Verification items for the finished model (mm, model axes). A direction names the side the tool comes from. Coordinates: 2 decimals unless noted, no trailing zeros. Write item = value, one per line.
```python
from build123d import *

# Parameters (mm, degrees)
SKETCH_1_R           = 1.5
SKETCH_1_R_2         = 17.5
SKETCH_1_R_3         = 12
SKETCH_1_R_4         = 1.25
EXTRUDE_1_DEPTH      = 4
SKETCH_2_R           = 18.5
SKETCH_2_R_2         = 17.5
CUT_EXTRUDE_1_DEPTH  = 3
SKETCH_3_W           = 10
SKETCH_3_H           = 5
SKETCH_3_W_2         = 6
CUT_EXTRUDE_2_DEPTH  = 93.020070098
CUT_EXTRUDE_3_DEPTH  = 93.020070098
FILLET_2_R           = 2
SKETCH_6_R           = 1.25
CUT_EXTRUDE_5_DEPTH  = 10
SKETCH_7_R           = 1.65
CUT_EXTRUDE_6_DEPTH  = 10
SKETCH_9_R           = 1.65
CUT_EXTRUDE_7_DEPTH  = 10
SKETCH_10_R          = 17.5
SKETCH_10_R_2        = 10.270750689
CUT_EXTRUDE_8_DEPTH  = 2
SKETCH_11_R          = 1.5
CUT_EXTRUDE_9_DEPTH  = 10
SKETCH_12_R          = 1.525
CUT_EXTRUDE_10_DEPTH = 10


with BuildPart() as part:
    # 草图1 → 凸台-拉伸1 (new body)
    with BuildSketch(Plane.XY):
        with BuildLine():
            Line((-27.534883443, -40.634933888), (42.465116557, -40.634933888))
            ThreePointArc((42.465116557, -40.634933888), (48.890398145, -38.615583047), (55.528781273, -37.478089862))
            ThreePointArc((55.528781273, -37.478089862), (82.425879892, -6.10109544), (52.465116557, 22.365066112))
            Line((52.465116557, 22.365066112), (-37.534883443, 22.365066112))
            ThreePointArc((-37.534883443, 22.365066112), (-67.495646778, -6.10109544), (-40.598548158, -37.478089862))
            ThreePointArc((-40.598548158, -37.478089862), (-33.960165031, -38.615583047), (-27.534883443, -40.634933888))
        make_face()
        with Locations((52.465116557, 13.115066112)):
            Circle(SKETCH_1_R, mode=Mode.SUBTRACT)
        with Locations((67.137582267, 7.037531822)):
            Circle(SKETCH_1_R, mode=Mode.SUBTRACT)
        with Locations((73.215116557, -7.634933888)):
            Circle(SKETCH_1_R, mode=Mode.SUBTRACT)
        with Locations((67.137582267, -22.307399597)):
            Circle(SKETCH_1_R, mode=Mode.SUBTRACT)
        with Locations((52.465116557, -28.384933888)):
            Circle(SKETCH_1_R, mode=Mode.SUBTRACT)
        with Locations((37.792650848, -22.307399597)):
            Circle(SKETCH_1_R, mode=Mode.SUBTRACT)
        with Locations((31.715116557, -7.634933888)):
            Circle(SKETCH_1_R, mode=Mode.SUBTRACT)
        with Locations((37.792650848, 7.037531822)):
            Circle(SKETCH_1_R, mode=Mode.SUBTRACT)
        with Locations(Location((-22.862417733, 7.037531822, 0), (0, 0, 180))):
            Circle(SKETCH_1_R, mode=Mode.SUBTRACT)
        with Locations(Location((-16.784883443, -7.634933888, 0), (0, 0, 180))):
            Circle(SKETCH_1_R, mode=Mode.SUBTRACT)
        with Locations(Location((-22.862417733, -22.307399597, 0), (0, 0, 180))):
            Circle(SKETCH_1_R, mode=Mode.SUBTRACT)
        with Locations(Location((-37.534883443, -28.384933888, 0), (0, 0, 180))):
            Circle(SKETCH_1_R, mode=Mode.SUBTRACT)
        with Locations(Location((-52.207349152, -22.307399597, 0), (0, 0, 180))):
            Circle(SKETCH_1_R, mode=Mode.SUBTRACT)
        with Locations(Location((-58.284883443, -7.634933888, 0), (0, 0, 180))):
            Circle(SKETCH_1_R, mode=Mode.SUBTRACT)
        with Locations(Location((-52.207349152, 7.037531822, 0), (0, 0, 180))):
            Circle(SKETCH_1_R, mode=Mode.SUBTRACT)
        with Locations(Location((-37.534883443, 13.115066112, 0), (0, 0, 180))):
            Circle(SKETCH_1_R, mode=Mode.SUBTRACT)
        with Locations((52.465116557, -7.634933888)):
            Circle(SKETCH_1_R_2, mode=Mode.SUBTRACT)
        with Locations(Location((-37.534883443, -7.634933888, 0), (0, 0, 180))):
            Circle(SKETCH_1_R_2, mode=Mode.SUBTRACT)
        with Locations((7.465116557, 2.365066112)):
            Circle(SKETCH_1_R_3, mode=Mode.SUBTRACT)
        with Locations((37.465116557, 19.365066112)):
            Circle(SKETCH_1_R, mode=Mode.SUBTRACT)
        with Locations((27.465116557, 19.365066112)):
            Circle(SKETCH_1_R, mode=Mode.SUBTRACT)
        with Locations(Location((-22.534883443, 19.365066112, 0), (0, 0, 180))):
            Circle(SKETCH_1_R, mode=Mode.SUBTRACT)
        with Locations(Location((-12.534883443, 19.365066112, 0), (0, 0, 180))):
            Circle(SKETCH_1_R, mode=Mode.SUBTRACT)
        with Locations((27.465116557, 2.365066112)):
            Circle(SKETCH_1_R_4, mode=Mode.SUBTRACT)
        with Locations(Location((-12.534883443, 2.365066112, 0), (0, 0, 180))):
            Circle(SKETCH_1_R_4, mode=Mode.SUBTRACT)
    extrude(amount=EXTRUDE_1_DEPTH)

    # 草图2 → 切除-拉伸1 (cut)
    # profile 1 of 2: a face of its own
    with BuildSketch(Plane.XY):
        with Locations((52.465116557, -7.634933888)):
            Circle(SKETCH_2_R)
        with Locations((52.465116557, -7.634933888)):
            Circle(SKETCH_2_R_2, mode=Mode.SUBTRACT)
    # profile 2 of 2: a face of its own
    with BuildSketch(Plane.XY):
        with Locations(Location((-37.534883443, -7.634933888, 0), (0, 0, 180))):
            Circle(SKETCH_2_R)
        with Locations(Location((-37.534883443, -7.634933888, 0), (0, 0, 180))):
            Circle(SKETCH_2_R_2, mode=Mode.SUBTRACT)
    extrude(amount=CUT_EXTRUDE_1_DEPTH, mode=Mode.SUBTRACT)

    # 草图3 → 切除-拉伸2 (cut, through all)
    with BuildSketch(Plane(origin=(0, 0, 0), x_dir=(-1, 0, 0), z_dir=(0, 0, -1))):
        with Locations((-27.465116557, -35.134933888)):
            Rectangle(SKETCH_3_W, SKETCH_3_H)
        with Locations((-10.465116557, -35.134933888)):
            Rectangle(SKETCH_3_W_2, SKETCH_3_H)
        with Locations((-4.465116557, -35.134933888)):
            Rectangle(SKETCH_3_W_2, SKETCH_3_H)
        with Locations((12.534883443, -35.134933888)):
            Rectangle(SKETCH_3_W, SKETCH_3_H)
    extrude(amount=-CUT_EXTRUDE_2_DEPTH, mode=Mode.SUBTRACT)

    # 草图4 → 切除-拉伸3 (cut, through all)
    with BuildSketch(Plane.XY.offset(4)):
        with BuildLine():
            Line((-5.446700673, -12.908603251), (-8.283381868, -15.745284446))
            ThreePointArc((-8.283381868, -15.745284446), (-3.541787321, -18.962101234), (1.82717455, -20.963320243))
            Line((1.82717455, -20.963320243), (2.862828881, -17.098205662))
            ThreePointArc((2.862828881, -17.098205662), (-1.539002487, -15.493428792), (-5.446700673, -12.908603251))
        make_face()
        with BuildLine():
            Line((20.391590305, -12.896201085), (23.228082643, -15.732693423))
            ThreePointArc((23.228082643, -15.732693423), (18.476716566, -18.959676916), (13.094689736, -20.96534121))
            Line((13.094689736, -20.96534121), (12.059024323, -17.100185272))
            ThreePointArc((12.059024323, -17.100185272), (16.473962924, -15.491044526), (20.391590305, -12.896201085))
        make_face()
        with BuildLine():
            Line((24.9885745, 12.005004999), (28.281142659, 14.310486044))
            ThreePointArc((28.281142659, 14.310486044), (30.089876696, 10.372576877), (31.161002411, 6.173608298))
            Line((31.161002411, 6.173608298), (27.272825293, 5.131774379))
            ThreePointArc((27.272825293, 5.131774379), (26.444429669, 8.672654702), (24.9885745, 12.005004999))
        make_face()
        with BuildLine():
            Line((-10.050135089, 12.019907372), (-13.342451817, 14.325212363))
            ThreePointArc((-13.342451817, 14.325212363), (-15.15680913, 10.380580957), (-16.230769297, 6.173608298))
            Line((-16.230769297, 6.173608298), (-12.342592179, 5.131774379))
            ThreePointArc((-12.342592179, 5.131774379), (-11.511512147, 8.680726255), (-10.050135089, 12.019907372))
        make_face()
    extrude(amount=-CUT_EXTRUDE_3_DEPTH, mode=Mode.SUBTRACT)

    # 圆角2
    fillet_2_edges = [part.edges().sort_by_distance(p)[0] for p in [
        (-10.050135089, 12.019907372, 2),
        (-12.342592179, 5.131774379, 2),
        (-16.230769297, 6.173608298, 2),
        (-13.342451817, 14.325212363, 2),
        (-5.446700673, -12.908603251, 2),
        (-8.283381868, -15.745284446, 2),
        (24.9885745, 12.005004999, 2),
        (27.272825293, 5.131774379, 2),
        (31.161002411, 6.173608298, 2),
        (28.281142659, 14.310486044, 2),
        (23.228082643, -15.732693423, 2),
        (20.391590305, -12.896201085, 2),
        (13.094689736, -20.96534121, 2),
        (12.059024323, -17.100185272, 2),
        (2.862828881, -17.098205662, 2),
        (1.82717455, -20.963320243, 2),
    ]]
    fillet(fillet_2_edges, radius=FILLET_2_R - 0.0001)  # a hair under: the kernel refuses the full size

    # 草图6 → 切除-拉伸5 (cut)
    with BuildSketch(Plane.XY.offset(4)):
        with Locations((-12.534883443, -20.571755315)):
            Circle(SKETCH_6_R)
        with Locations((27.465116557, -20.571755315)):
            Circle(SKETCH_6_R)
    extrude(amount=-CUT_EXTRUDE_5_DEPTH, mode=Mode.SUBTRACT)

    # 草图7 → 切除-拉伸6 (cut)
    with BuildSketch(Plane.XY.offset(4)):
        with Locations((43.683121449, -35.634933888)):
            Circle(SKETCH_7_R)
        with Locations((63.683121449, -31.634933888)):
            Circle(SKETCH_7_R)
        with Locations((-48.752888335, -31.634933888)):
            Circle(SKETCH_7_R)
        with Locations((-28.752888335, -35.634933888)):
            Circle(SKETCH_7_R)
    extrude(amount=-CUT_EXTRUDE_6_DEPTH, mode=Mode.SUBTRACT)

    # 草图9 → 切除-拉伸7 (cut)
    with BuildSketch(Plane.XY.offset(4)):
        with Locations((7.465116557, 17.365066112)):
            Circle(SKETCH_9_R)
        with Locations((20.455497614, 9.865066112)):
            Circle(SKETCH_9_R)
        with Locations((20.455497614, -5.134933888)):
            Circle(SKETCH_9_R)
        with Locations((7.465116557, -12.634933888)):
            Circle(SKETCH_9_R)
        with Locations((-5.5252645, -5.134933888)):
            Circle(SKETCH_9_R)
        with Locations((-5.5252645, 9.865066112)):
            Circle(SKETCH_9_R)
    extrude(amount=-CUT_EXTRUDE_7_DEPTH, mode=Mode.SUBTRACT)

    # 草图10 → 切除-拉伸8 (cut)
    with BuildSketch(Plane.XY):
        with Locations((7.465116557, 2.365066112)):
            Circle(SKETCH_10_R)
        with Locations((7.465116557, 2.365066112)):
            Circle(SKETCH_10_R_2, mode=Mode.SUBTRACT)
    extrude(amount=CUT_EXTRUDE_8_DEPTH, mode=Mode.SUBTRACT)

    # 草图11 → 切除-拉伸9 (cut)
    with BuildSketch(Plane.XY.offset(4)):
        with Locations((17.465116557, -29.634933888)):
            Circle(SKETCH_11_R)
        with Locations((27.465116557, -29.634933888)):
            Circle(SKETCH_11_R)
        with Locations((-12.534883443, -29.634933888)):
            Circle(SKETCH_11_R)
        with Locations((-2.534883443, -29.634933888)):
            Circle(SKETCH_11_R)
    extrude(amount=-CUT_EXTRUDE_9_DEPTH, mode=Mode.SUBTRACT)

    # 草图12 → 切除-拉伸10 (cut)
    with BuildSketch(Plane(origin=(0, 0, 0), x_dir=(-1, 0, 0), z_dir=(0, 0, -1))):
        with Locations((39.752888335, -34.034253729)):
            Circle(SKETCH_12_R)
        with Locations((54.752888335, -27.769082524)):
            Circle(SKETCH_12_R)
        with Locations(Location((-69.683121449, -27.769082524, 0), (0, 0, 180))):
            Circle(SKETCH_12_R)
        with Locations(Location((-54.683121449, -34.034253729, 0), (0, 0, 180))):
            Circle(SKETCH_12_R)
    extrude(amount=-CUT_EXTRUDE_10_DEPTH, mode=Mode.SUBTRACT)


solid = part.part
```
Item 1: Scan lines: L1, parallel to Y at x = -17, z = 3.3; L2, parallel to Y at x = 65, z = 1.95; L3, parallel to Y at x = -53.5, z = 3.35. Record each from-to range of solid material in increasing order. Write a range as from..to.
Report:
L1 = -40.63..-37.63, -32.63..-9.12, -6.15..22.37
L2 = -34.89..-32.63, -30.64..-21.24, 5.97..19.62
L3 = -33.03..-28.64, -26.9..-23.07, -21.55..-14.8, -0.47..6.28, 7.8..17.76
Item 2: Tool access check on faces 3 (the cylindrical face through (-10.685, 11.92, 1.972)), 4 (the flat face through (-26, 6, 3)). Record the directions out of +Z, -Z, +X, -X, +Y, -Y that give a thin tool (end or side, any length) a straight path to the whole face; none if there is none.
Report:
face_3 = +Z, -Z
face_4 = -Z
Item 3: Release check for a two-part mould opening along X. For faces 1 (the cylindrical face through (-38.966, 12.665, 1.972)), 2 (the flat face through (8, 22.365, 2)) record: pulls with the +X half, pulls with the -X half, needs draft (parallel to the pull), parting line crosses it, or undercut.
Report:
face_1 = undercut
face_2 = needs draft
Item 4: Sectioned sample at A-A, the plane z = 1. Give the number of separate pieces and of enclosed holes in the cut face, then the cut area to 3 significant figures.
Report:
separate_pieces = 1
enclosed_holes = 46
area = 4,810 mm^2
